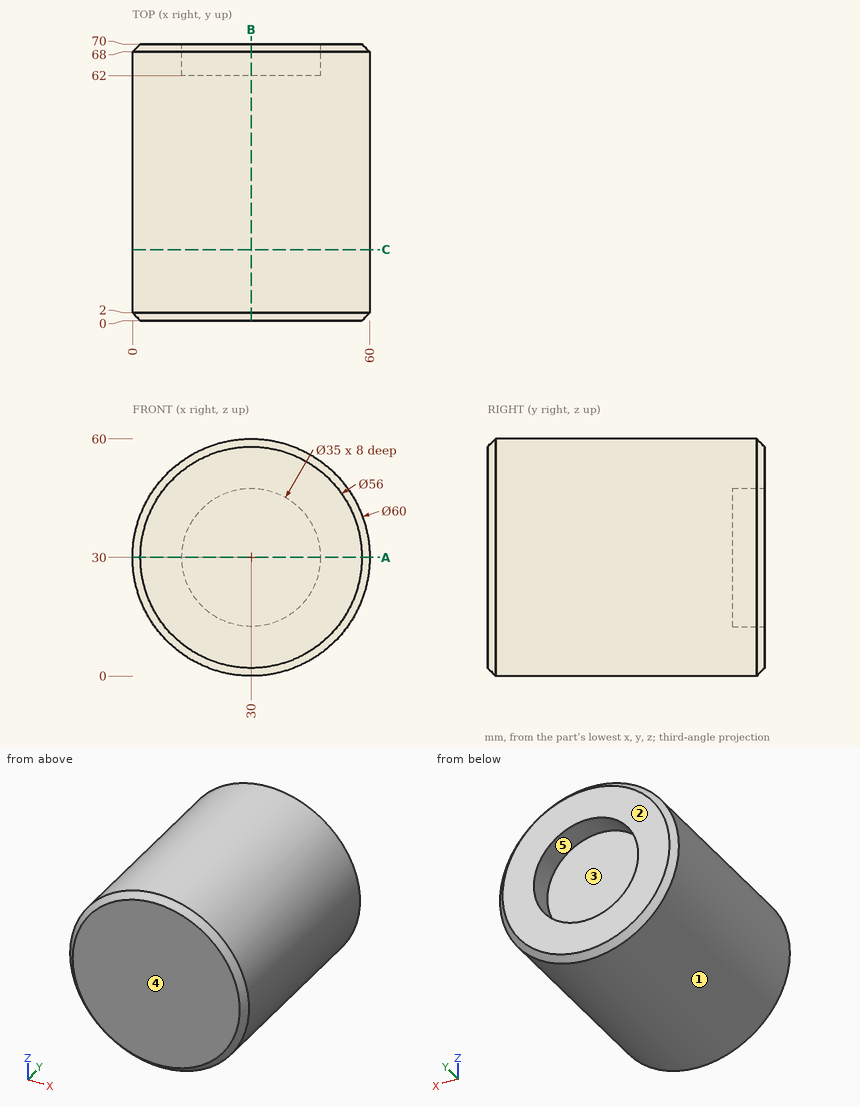
Geometry: see drawing. Coordinates: mm, zero at the bounding-box minimum. A direction names the side the tool comes from. Round coordinates to 2 decimals unless told otherwise and drop trailing zeros. Loops run counter-clockwise (first coordinate to the right, second up) from the corner with the lowest first, then second, coordinate; pieces in that order, holes last. Notation, with made-up numbers: (-33, 51.5) -> (25, 51.5) arc R32 ccw to (25, 85.5) -> close; hole circle Ø3 at (66.25, 66.5). An arc over 180 degrees is marked (long way). Use one line per item in the form item = value. Start each with the question number.
Item 1: Set-up query: the marked faces 4 and 5. Return all of +Z, -Z, +X, -X, +Y, -Y with unobstructed straight access to the full face (end or side cutting, diameter ignored); none if empty.
Item 2: Section query A-A on z = 30. Return the cut outline in (x, y), then the cut area to 3 significant figures.
Item 3: Mould query, pull axis X, two halves, no side actions, for the marked faces 1, 2 and 3. Classes: pulls with the +X half, pulls with the -X half, needs draft (parallel to the pull), parting line crosses it, or undercut.
Item 4: Section query C-C on y = 18. Return the cut outline in (x, z).
Item 5: Section query B-B on x = 30. Return the cut outline in (y, z).
Item 6: Contact query for flat-ended pins moving along their axis: pin 1 Ø6 at (x, y) = (49.5, 45.5) entering from -Z; pin 2 Ø8 at (y, z) = (20.5, 49.5) entering from -X; pin 3 Ø1 at (y, z) = (10, 18) entering from +X. Output: stop coordinate, or through.
Item 7: Material intervals for L1, parallel to X at y = 28.5, z = 29; L2, parallel to Y at x = 31, z = 23; L3, parallel to Z at x = 30, y = 67, sorted ascending. Write a range as from..to.
Ans:
q1.face_4 = +Z, -Z, +X, -X, -Y
q1.face_5 = +Y
q2.outline = (0, 2) -> (2, 0) -> (58, 0) -> (60, 2) -> (60, 68) -> (58, 70) -> (47.5, 70) -> (47.5, 62) -> (12.5, 62) -> (12.5, 70) -> (2, 70) -> (0, 68) -> close
q2.area = 3,910 mm^2
q3.face_1 = parting line crosses it
q3.face_2 = needs draft
q3.face_3 = undercut
q4.outline = circle Ø60 at (30, 30)
q5.outline = (0, 2) -> (2, 0) -> (68, 0) -> (70, 2) -> (70, 12.5) -> (62, 12.5) -> (62, 47.5) -> (70, 47.5) -> (70, 58) -> (68, 60) -> (2, 60) -> (0, 58) -> close
q6.pin_1 = 4.95
q6.pin_2 = 4.31
q6.pin_3 = 57.71
q7.L1 = 0.02..59.98
q7.L2 = 0..62
q7.L3 = 0..12.5, 47.5..60
